Input: part model. Units: mm. Frame: model coordinates. A direction names the side the tool comes from. Give positions to 0.01 mm unless a question says otherwise; leave off trailing zeros. Write each loop counter-clockwise with the first axis right and the second up, starting at its lowest first coordinate (ties: lowest second). Pieces come first, ordered by that corner, then holes. Notation, with made-up numbers: (-16, 73.5) - (18, 73.5) arc R22 cw to (18, 80.5) - close; hole circle Ø7 at (-29, 41). An arc over 180 degrees is marked (long way). Use a Markdown table: item, result. Add a question column.
1. Set-up query: faces 1 (the flat face through (4.507, -3.538, 4.93)), 2 (the flat face through (3.125, 6, 5)), 3 (the flat face through (4, -4, 5)). Return all of +Z, -Z, +X, -X, +Y, -Y with unobstructed straight access to the full face (end or side cutting, diameter ignored); none if empty.
2. Section query A-A, the plane y = -3.75. Return loops of the section in (x, z).
3. Section query C-C, the plane y = 2.75. Return loops of the section in (x, z), plus the area to 3 significant figures.
4. Pin query (flat end, axial travel): pin 1 (0.6 mm diameter, centred on x = 3.5, z = 6, fed in from -Y); pin 2 (1 mm diameter, centred on x = -5, z = 7, fed in from +Y); pin 3 (1.2 mm diameter, centred on y = 6, z = 5.5, fed in from -X) (3 decimals). Return the tip coordinate at first contact, or that it passes through.
5. Material intervals for probe 1 along X at (y, z) = (-2, 9.5); probe 2 along Y at (x, z) = (2.75, 6.25); probe 3 along Y at (x, z) = (-6, 5.5), sorted ascending.
6. Mould query, pull axis Y, two halves, no side actions, for faces 4 (the flat face through (-5, -5, 5)), 5 (the flat face through (-3.125, 6, 5)), 6 (the flat face through (-4, -4, 5)). Classes: released by +Y, released by -Y, zero draft, split by the parting line, or undercut.
7. Section query B-B, the plane z = 3. Return loops of the section in (x, y) (3 decimals).
8. Section query D-D, the plane y = 8. Return loops of the section in (x, z).
```python
from build123d import *

# Parameters (mm, degrees)
F1_DEPTH = 10


with BuildPart() as f1:
    # F0 (on Top) → F1 (new body)
    with BuildSketch(Plane.XY):
        with BuildLine():
            Line((-6.5, -5), (-4, -5))
            Line((-4, -5), (-4, -3.576375))
            Line((-4, -3.576375), (-5, -3.5))
            Line((-5, -3.5), (-5, 3.5))
            Line((-5, 3.5), (5, 3.5))
            Line((5, 3.5), (5, -3.5))
            Line((5, -3.5), (4, -3.576375))
            Line((4, -3.576375), (4, -5))
            Line((4, -5), (6.5, -5))
            Line((6.5, -5), (6.5, 5))
            Line((6.5, 5), (3.125, 5))
            Line((3.125, 5), (3.125, 7.5))
            Line((3.125, 7.5), (3.627, 7.5))
            ThreePointArc((3.627, 7.5), (4.127, 8), (3.627, 8.5))
            Line((3.627, 8.5), (-3.627, 8.5))
            ThreePointArc((-3.627, 8.5), (-4.127, 8), (-3.627, 7.5))
            Line((-3.627, 7.5), (-3.125, 7.5))
            Line((-3.125, 7.5), (-3.125, 5))
            Line((-3.125, 5), (-6.5, 5))
            Line((-6.5, 5), (-6.5, -5))
        make_face()
    extrude(amount=F1_DEPTH)


solid = f1.part
```
Result sheet:
| question | item | result |
|---|---|---|
| 1 | face 1 | +Z, -Z |
| 1 | face 2 | +Z, -Z, +X |
| 1 | face 3 | +Z, -Z, -Y |
| 2 | outline | (-6.5, 0) - (-4, 0) - (-4, 10) - (-6.5, 10) - close; (4, 0) - (6.5, 0) - (6.5, 10) - (4, 10) - close |
| 3 | outline | (-6.5, 0) - (-5, 0) - (-5, 10) - (-6.5, 10) - close; (5, 0) - (6.5, 0) - (6.5, 10) - (5, 10) - close |
| 3 | area | 30.0 mm² |
| 4 | pin 1 | stops at y = 3.5 |
| 4 | pin 2 | stops at y = 5 |
| 4 | pin 3 | stops at x = -3.125 |
| 5 | probe 1 | x = -6.5 to -5, 5 to 6.5 |
| 5 | probe 2 | y = 3.5 to 8.5 |
| 5 | probe 3 | y = -5 to 5 |
| 6 | face 4 | released by -Y |
| 6 | face 5 | undercut |
| 6 | face 6 | zero draft |
| 7 | outline | (-6.5, -5) - (-4, -5) - (-4, -3.576) - (-5, -3.5) - (-5, 3.5) - (5, 3.5) - (5, -3.5) - (4, -3.576) - (4, -5) - (6.5, -5) - (6.5, 5) - (3.125, 5) - (3.125, 7.5) - (3.627, 7.5) arc R0.5 ccw to (3.627, 8.5) - (-3.627, 8.5) arc R0.5 ccw to (-3.627, 7.5) - (-3.125, 7.5) - (-3.125, 5) - (-6.5, 5) - close |
| 8 | outline | (-4.13, 0) - (4.13, 0) - (4.13, 10) - (-4.13, 10) - close |
